from build123d import *

# Parameters (mm, degrees)
EXTRUSION1_DEPTH = 1


with BuildPart() as part:
    # Esquisse1 → Extrusion1 (new body)
    with BuildSketch(Plane.XY):
        with BuildLine():
            Line((5.45058398, -1.312131796), (4.907576652, -2.710396092))
            ThreePointArc((4.907576652, -2.710396092), (5.320441767, -3.72745699), (6.359982311, -3.375))
            ThreePointArc((6.359982311, -3.375), (0, 7.2), (-6.359982311, -3.375))
            ThreePointArc((-6.359982311, -3.375), (-5.320441767, -3.72745699), (-4.907576652, -2.710396092))
            Line((-4.907576652, -2.710396092), (-5.45058398, -1.312131796))
            ThreePointArc((-5.45058398, -1.312131796), (-5.58638878, -1.084069901), (-5.789339137, -0.91299587))
            ThreePointArc((-5.789339137, -0.91299587), (-6.103454982, -0.570684122), (-6.174372427, -0.111536201))
            ThreePointArc((-6.174372427, -0.111536201), (-4.07266037, 3.620779969), (0, 4.947737042))
            ThreePointArc((0, 4.947737042), (4.07266037, 3.620779969), (6.174372427, -0.111536201))
            ThreePointArc((6.174372427, -0.111536201), (6.103454982, -0.570684122), (5.789339137, -0.91299587))
            ThreePointArc((5.789339137, -0.91299587), (5.58638878, -1.084069901), (5.45058398, -1.312131796))
        make_face()
    extrude(amount=EXTRUSION1_DEPTH)


solid = part.part
Verification items for the finished model (mm, model axes). A direction names the side the tool comes from. Give positions to 0.01 mm unless a question says otherwise; leave off trailing zeros. Loops run counter-clockwise (first coordinate to the right, second up) from the corner with the lowest first, then second, coordinate; pieces in that order, holes last.
1) Thickness scan on line 1 along X through (y, z) = (-1.75, 0.2); line 2 along X through (y, z) = (2.25, 0.1); line 3 along Y through (x, z) = (-5.5, 0.9). Record the ranges inside material, lowest first.
2) Sectioned sample at A-A, the plane y = -3. Enter the section's corners in (x, z).
3) Sectioned sample at C-C, the plane y = 0.5. Enter the section's corners in (x, z).
4) Draft check along X on faces 1 (the flat face through (-1.1, 5.4, 1)), 2 (the cylindrical face through (-4.1, 3.6, 0.5)), 3 (the flat face through (-5.175, -2.021, 0.493)), 4 (the cylindrical face through (0.207, 7.197, 0.493)). Enter one of: pulls with the +X half, pulls with the -X half, needs draft (parallel to the pull), parting line crosses it, or undercut.
5) Set-up check for faces 5 (the flat face through (5.183, -2.001, 0.493)), 6 (the flat face through (-1.1, 5.4, 0)): record each of +Z, -Z, +X, -X, +Y, -Y from which the full face is reachable in a straight line by a thin tool's end or side.
6) Depth check by flat-ended pin: pin 1 Ø3 at (x, y) = (3.5, 1) entering from -Z. Enter the tip coordinate at first touch or a pass-through.
7) Sectioned sample at B-B, the plane z = 0.45. Enter the section's corners in (x, y) (3 decimals).
8) Sectioned sample at D-D, the plane x = 3.75. Enter the section's corners in (y, z).
Answers:
1. line 1: x = -6.98 to -5.28, 5.28 to 6.98
1. line 2: x = -6.84 to -5.29, 5.29 to 6.84
1. line 3: y = -3.79 to -1.21, 1.91 to 4.65
2. outline: (-6.55, 0) - (-4.85, 0) - (-4.85, 1) - (-6.55, 1) - close; (4.85, 0) - (6.55, 0) - (6.55, 1) - (4.85, 1) - close
3. outline: (-7.18, 0) - (-6.05, 0) - (-6.05, 1) - (-7.18, 1) - close; (6.05, 0) - (7.18, 0) - (7.18, 1) - (6.05, 1) - close
4. face 1: needs draft
4. face 2: undercut
4. face 3: undercut
4. face 4: parting line crosses it
5. face 5: +Z, -Z
5. face 6: -Z, +X, -X, +Y, -Y
6. pin 1: passes through
7. outline: (-6.36, -3.375) arc R0.8 ccw to (-4.908, -2.71) - (-5.451, -1.312) arc R0.8 ccw to (-5.789, -0.913) arc R0.8 cw to (-6.174, -0.112) arc R5.9 cw to (0, 4.948) arc R5.9 cw to (6.174, -0.112) arc R0.8 cw to (5.789, -0.913) arc R0.8 ccw to (5.451, -1.312) - (4.908, -2.71) arc R0.8 ccw to (6.36, -3.375) arc R7.2 ccw (long way) to start
8. outline: (3.87, 0) - (6.15, 0) - (6.15, 1) - (3.87, 1) - close
